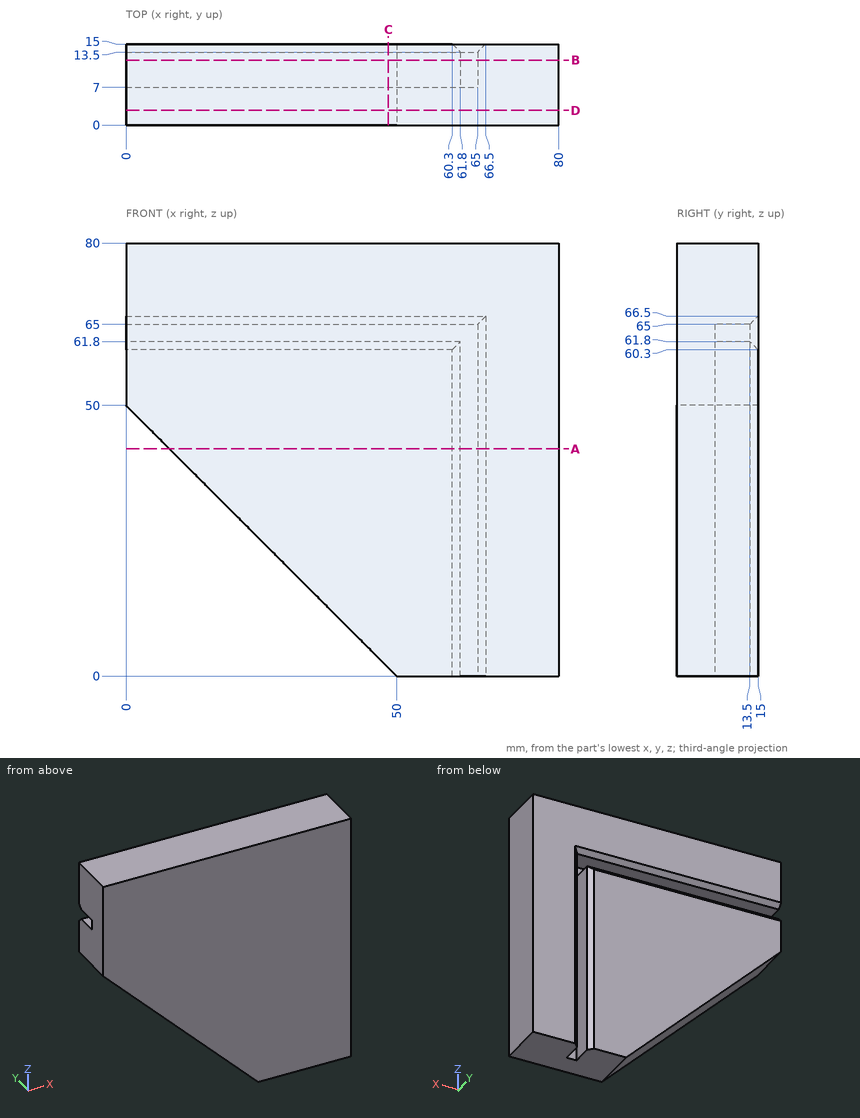
Input: dimensioned drawing with shaded views. Units: mm. Origin: part minimum x, y, z. Round coordinates to 2 decimals unless told otherwise and drop trailing zeros. Order: outer loops, then holes, each group sorted by start corner. A loop starts at its lowest first (then second) coordinate and runs counter-clockwise, first axis right, second up. Notation, with made-up numbers: M 47,63.5 L 54,63.5 A22 ccw 54,100.5 Z; hole C -35,65 d2. An arc over 180 degrees is marked long. Use one line per item in the form item = value. Start each with the question number.
Q1. Material intervals for line 1 (X direction, y = 13, z = 54.5); line 2 (Y direction, x = 63.5, z = 63); line 3 (Z direction, x = 35, y = 14.5), sorted ascending. Write a range as [from, to].
Q2. Pin query (flat end, axial travel): pin 1 Ø4 at (x, y) = (52, 6) entering from -Z; pin 2 Ø2 at (y, z) = (9, 39) entering from -X; pin 3 Ø2 at (x, y) = (18, 9.5) entering from -Z. Return the tip coordinate at first contact, or that it passes through.
Q3. Cut plane A-A (z = 42). Return loops of the section in (x, y).
Q4. Cut plane C-C (x = 48.5). Return loops of the section in (y, z).
Q5. Cut plane D-D (y = 2.75). Return loops of the section in (x, z).
Q6. Cut plane B-B (y = 12). Return loops of the section in (x, z), and give its area (3 significant figures).
Geometry results:
q1.line_1 = [0, 61.8], [65, 80]
q1.line_2 = [0, 7]
q1.line_3 = [15, 60.8], [66, 80]
q2.pin_1 = 0
q2.pin_2 = 10
q2.pin_3 = 31
q3.outline = M 8,0 L 80,0 L 80,15 L 66.5,15 L 65,13.5 L 65,7 L 61.8,7 L 61.8,13.5 L 60.3,15 L 8,15 Z
q4.outline = M 0,1.5 L 15,1.5 L 15,60.3 L 13.5,61.8 L 7,61.8 L 7,65 L 13.5,65 L 15,66.5 L 15,80 L 0,80 Z
q5.outline = M 0,50 L 50,0 L 80,0 L 80,80 L 0,80 Z
q6.outline = M 0,50 L 50,0 L 61.8,0 L 61.8,61.8 L 0,61.8 Z; M 0,65 L 65,65 L 65,0 L 80,0 L 80,80 L 0,80 Z
q6.area = 4,740 mm^2
